from build123d import *

# Parameters (mm, degrees)
SKETCH1_W     = 26.67
SKETCH1_H     = 1.27
CHAMFER1_SIZE = 1.25


with BuildPart() as part:
    # Sketch1 → Revolve1 (revolve)
    with BuildSketch(Plane.XY, mode=Mode.PRIVATE) as revolve1_sk:
        with Locations((13.335, 0.635)):
            Rectangle(SKETCH1_W, SKETCH1_H)
        with BuildLine():
            Line((3.18, 85.55), (0, 85.55))
            Line((0, 85.55), (0, 1.27))
            Line((0, 1.27), (26.67, 1.27))
            Line((26.67, 1.27), (24.76, 3.18))
            Line((24.76, 3.18), (18.43, 3.18))
            ThreePointArc((18.43, 3.18), (7.646621587, 7.646621587), (3.18, 18.43))
            Line((3.18, 18.43), (3.18, 85.55))
        make_face()
    revolve(revolve1_sk.sketch.rotate(Axis((0, 91.878860224, 0), (0, -1, 0)), 90), axis=Axis((0, 91.878860224, 0), (0, -1, 0)))

    # Chamfer1
    chamfer1_edges = [part.edges().sort_by_distance(p)[0] for p in [
        (0, 85.55, -3.18),
    ]]
    chamfer(chamfer1_edges, length=CHAMFER1_SIZE)


solid = part.part
Here's how the part is built. I have some questions about the finished solid (model axes, mm). A direction names the side the tool comes from. Round coordinates to 2 decimals unless told otherwise and drop trailing zeros. Order: outer loops, then holes, each group sorted by start corner. A loop starts at its lowest first (then second) coordinate and runs counter-clockwise, first axis right, second up. Notation, with made-up numbers: M -30.5,18 L 6.5,18 A9 ccw 6.5,28 Z; hole C 59,63 d5. An arc over 180 degrees is marked long. Return JSON: item names as keys, results as strings. Group by question number.
1. If we section it at D-D on y = 13: List the corners of the cut face in (x, z) for me.
2. If we section it at C-C on y = 77.5: List the corners of the cut face in (x, z) for me.
3. I'm going to push flat-ended pins straight in: pin 1 Ø6 at (y, z) = (34.5, -5) entering from -X; pin 2 Ø5 at (x, y) = (2.5, 39.5) entering from +Z; pin 3 Ø1 at (y, z) = (35.5, 5) entering from -X; pin 4 Ø6 at (y, z) = (36.5, 4.5) entering from -X. Where does each tip first touch, or does it pass through?
4. Please list where these lines run through material, in increasing order: probe 1 along Y at (x, z) = (18.5, -7.5); probe 2 along Y at (x, z) = (4.5, 3.5); probe 3 along X at (y, z) = (51, 1).
5. If we section it at B-B on z = 0: List the corners of the cut face in (x, y) for me, then the cut area to 3 significant figures.
6. On a 3-axis mill with a long thin cutter (end or side, diameter ignored), from which of +Z, -Z, +X, -X, +Y, -Y can I reach the whole of each face in a straight line? I mean faces 1 (the face through (-26.443, 0.644, -3.472)), 2 (the face through (1.935, 51.826, -2.524)). Say none if no direction works.
7. If we section it at A-A on x = 0: List the corners of the cut face in (y, z) for me, then the cut area to 3 significant figures.
Reply:
{
 "1": {"outline": "C 0,0 d8.36"},
 "2": {"outline": "C 0,0 d6.36"},
 "3": {"pin 1": "x = -2.47", "pin 2": "z = 3.18", "pin 3": "through", "pin 4": "x = -2.8"},
 "4": {"probe 1": "0 to 3.18", "probe 2": "0 to 10.03", "probe 3": "-3.02 to 3.02"},
 "5": {"outline": "M -26.67,0 L 26.67,0 L 26.67,1.27 L 24.76,3.18 L 18.43,3.18 A15.25 cw 3.18,18.43 L 3.18,84.3 L 1.93,85.55 L -1.93,85.55 L -3.18,84.3 L -3.18,18.43 A15.25 cw -18.43,3.18 L -24.76,3.18 L -26.67,1.27 Z", "area": "788 mm^2"},
 "6": {"face 1": "+Y, -Y", "face 2": "+Y"},
 "7": {"outline": "M 0,-26.67 L 1.27,-26.67 L 3.18,-24.76 L 3.18,-18.43 A15.25 cw 18.43,-3.18 L 84.3,-3.18 L 85.55,-1.93 L 85.55,1.93 L 84.3,3.18 L 18.43,3.18 A15.25 cw 3.18,18.43 L 3.18,24.76 L 1.27,26.67 L 0,26.67 Z", "area": "788 mm^2"}
}
